Autodesk Inventor part; units mm, degrees
ref_plane "YZ Plane" through (0, 0, 0) normal (1, 0, 0) x (0, 1, 0)
ref_plane "XZ Plane" through (0, 0, 0) normal (0, 1, 0) x (-1, 0, 0)
ref_plane "XY Plane" through (0, 0, 0) normal (0, 0, 1) x (1, 0, 0)
sketch "Boceto1" plane through (0, 0, 0) normal (0, 0, 1) x (1, 0, 0)
  line L0 (0, 71.5) -> (84.4, 71.5)
  line L1 (0, 0) -> (4.5, 0)
  line L2 (62.2, 0) -> (62.2, 35)
  line L3 (62.2, 35) -> (112.2, 35)
  line L4 (112.2, 35) -> (112.2, 0)
  line L5 (84.4, 58.5) -> (84.4, 71.5)
  line L6 (84.4, 58.5) -> (0, 58.5)
  line L7 (87.2, 35) -> (108.2, 35)
  circle A0 centre (108.2, 46.75) radius 1.65
  circle A1 centre (66.2, 46.75) radius 1.65
  circle A2 centre (31.1, 43.75) radius 3
  circle A3 centre (178.7, 0) radius 2.5
  circle A4 centre (68.5, 81.35) radius 1.65
  line L8 (0, 90) -> (105.7, 90)
  arc A5 (120.7782, 83.1308) -> (105.7, 90) centre (105.672, 69.9553) ccw
  line L9 (200, 0) -> (200, 30.4)
  arc A6 (200, 30.4) -> (192, 38.4) centre (192, 30.4) ccw
  arc A7 (120.7782, 83.1308) -> (192, 38.4) centre (202.3119, 133.8853) ccw
  line L10 (4.5, 80.75) -> (4.5, 85.3)
  line L11 (4.5, 85.3) -> (0, 82.7)
  line L12 (4.5, 80.75) -> (4.5, 76.2)
  line L13 (4.5, 76.2) -> (0, 78.8)
  line L14 (0, 90) -> (0, 82.7)
  line L15 (0, 58.5) -> (0, 53.5)
  line L16 (0, 48.4) -> (0, 46.75)
  line L17 (0, 78.8) -> (0, 71.5)
  line L18 (0, 58.5) -> (0, 53.5)
  line L19 (0, 53.5) -> (0, 48.4)
  line L20 (0, 58.5) -> (0, 37.5)
  line L21 (9.1, 34.95) -> (9.1, 41.75)
  line L22 (9.1, 41.75) -> (0, 37.5)
  line L23 (9.1, 34.95) -> (9.1, 28.15)
  line L24 (9.1, 28.15) -> (0, 32.4)
  line L25 (0, 0) -> (0, 32.4)
  line L26 (0, 37.5) -> (0, 46.75)
  line L27 (0, -71.5) -> (84.4, -71.5)
  line L28 (62.2, 0) -> (62.2, -35)
  line L29 (62.2, -35) -> (112.2, -35)
  line L30 (112.2, -35) -> (112.2, 0)
  line L31 (84.4, -58.5) -> (84.4, -71.5)
  line L32 (84.4, -58.5) -> (0, -58.5)
  line L33 (87.2, -35) -> (108.2, -35)
  circle A8 centre (108.2, -46.75) radius 1.65
  circle A9 centre (66.2, -46.75) radius 1.65
  circle A10 centre (31.1, -43.75) radius 3
  circle A11 centre (178.7, 0) radius 2.5
  circle A12 centre (68.5, -81.35) radius 1.65
  line L34 (0, -90) -> (105.7, -90)
  arc A13 (105.7, -90) -> (120.7782, -83.1308) centre (105.672, -69.9553) ccw
  line L35 (200, 0) -> (200, -30.4)
  arc A14 (192, -38.4) -> (200, -30.4) centre (192, -30.4) ccw
  arc A15 (192, -38.4) -> (120.7782, -83.1308) centre (202.3119, -133.8853) ccw
  line L36 (4.5, -80.75) -> (4.5, -85.3)
  line L37 (4.5, -85.3) -> (0, -82.7)
  line L38 (4.5, -80.75) -> (4.5, -76.2)
  line L39 (4.5, -76.2) -> (0, -78.8)
  line L40 (0, -90) -> (0, -82.7)
  line L41 (0, -58.5) -> (0, -53.5)
  line L42 (0, -48.4) -> (0, -46.75)
  line L43 (0, -78.8) -> (0, -71.5)
  line L44 (0, -58.5) -> (0, -53.5)
  line L45 (0, -53.5) -> (0, -48.4)
  line L46 (0, -58.5) -> (0, -37.5)
  line L47 (9.1, -34.95) -> (9.1, -41.75)
  line L48 (9.1, -41.75) -> (0, -37.5)
  line L49 (9.1, -34.95) -> (9.1, -28.15)
  line L50 (9.1, -28.15) -> (0, -32.4)
  line L51 (0, 0) -> (0, -32.4)
  line L52 (0, -37.5) -> (0, -46.75)
  line L53 (261.8168, 58.5) -> (321.3628, 58.5)
  line L54 (321.3628, 58.5) -> (321.3628, -17.5)
  line L55 (321.3628, -17.5) -> (261.8168, -17.5)
  line L56 (261.8168, -17.5) -> (261.8168, 58.5)
sketch "Boceto3" plane through (0, 0, 0) normal (0, 0, 1) x (1, 0, 0)
  line L0 (-258.9506, 92.2639) -> (-258.9506, 96.8139)
  line L1 (-258.9506, 96.8139) -> (-263.4506, 94.2139)
  line L2 (-258.9506, 92.2639) -> (-258.9506, 87.7139)
  line L3 (-258.9506, 87.7139) -> (-263.4506, 90.3139)
  line L4 (-263.4506, 101.5139) -> (-263.4506, 94.2139)
  line L5 (-263.4506, 70.0139) -> (-263.4506, 65.0139)
  line L6 (-263.4506, 59.9139) -> (-263.4506, 58.2639)
  line L7 (-263.4506, 90.3139) -> (-263.4506, 83.0139)
  line L8 (-263.4506, 70.0139) -> (-263.4506, 65.0139)
  line L9 (-263.4506, 65.0139) -> (-263.4506, 59.9139)
  line L10 (-263.4506, 70.0139) -> (-263.4506, 49.0139)
  line L11 (-254.3506, 46.4639) -> (-254.3506, 53.2639)
  line L12 (-254.3506, 53.2639) -> (-263.4506, 49.0139)
  line L13 (-254.3506, 46.4639) -> (-254.3506, 39.6639)
  line L14 (-254.3506, 39.6639) -> (-263.4506, 43.9139)
  line L15 (-263.4506, 11.5139) -> (-263.4506, 43.9139)
  line L16 (-263.4506, 49.0139) -> (-263.4506, 58.2639)
  line L17 (-263.4506, 83.0139) -> (-322.4506, 83.0139)
  line L18 (-263.4506, 83.0139) -> (-322.4506, 83.0139)
  line L19 (-263.4506, 70.0139) -> (-322.4506, 70.0139)
  line L20 (-322.4506, 70.0139) -> (-322.4506, 83.0139)
  circle A0 centre (-322.4506, 55.4139) radius 3
  line L21 (-350.4506, 83.0139) -> (-350.4506, 93.5139)
  circle A1 centre (-272.1006, 92.8639) radius 1.65
  line L22 (-342.4506, 101.5139) -> (-263.4506, 101.5139)
  line L23 (-373.8506, 11.5139) -> (-373.8506, 24.6339)
  arc A2 (-368.1081, 32.3088) -> (-373.8506, 24.6339) centre (-365.8506, 24.6339) ccw
  arc A3 (-342.4506, 101.5139) -> (-350.4506, 93.5139) centre (-342.4506, 93.5139) ccw
  arc A4 (-368.1081, 32.3088) -> (-350.4675, 52.85) centre (-376.4854, 57.3485) ccw
  line L24 (-350.4506, 83.0139) -> (-350.4506, 53.0604)
  arc A5 (-350.4675, 52.85) -> (-350.4506, 53.0604) centre (-357.2375, 53.5013) ccw
  line L25 (-258.9506, -69.2361) -> (-258.9506, -73.7861)
  line L26 (-258.9506, -73.7861) -> (-263.4506, -71.1861)
  line L27 (-258.9506, -69.2361) -> (-258.9506, -64.6861)
  line L28 (-258.9506, -64.6861) -> (-263.4506, -67.2861)
  line L29 (-263.4506, -78.4861) -> (-263.4506, -71.1861)
  line L30 (-263.4506, -46.9861) -> (-263.4506, -41.9861)
  line L31 (-263.4506, -36.8861) -> (-263.4506, -35.2361)
  line L32 (-263.4506, -67.2861) -> (-263.4506, -59.9861)
  line L33 (-263.4506, -46.9861) -> (-263.4506, -41.9861)
  line L34 (-263.4506, -41.9861) -> (-263.4506, -36.8861)
  line L35 (-263.4506, -46.9861) -> (-263.4506, -25.9861)
  line L36 (-254.3506, -23.4361) -> (-254.3506, -30.2361)
  line L37 (-254.3506, -30.2361) -> (-263.4506, -25.9861)
  line L38 (-254.3506, -23.4361) -> (-254.3506, -16.6361)
  line L39 (-254.3506, -16.6361) -> (-263.4506, -20.8861)
  line L40 (-263.4506, 11.5139) -> (-263.4506, -20.8861)
  line L41 (-263.4506, -25.9861) -> (-263.4506, -35.2361)
  line L42 (-263.4506, -59.9861) -> (-322.4506, -59.9861)
  line L43 (-263.4506, -59.9861) -> (-322.4506, -59.9861)
  line L44 (-263.4506, -46.9861) -> (-322.4506, -46.9861)
  line L45 (-322.4506, -46.9861) -> (-322.4506, -59.9861)
  circle A6 centre (-322.4506, -32.3861) radius 3
  line L46 (-350.4506, -59.9861) -> (-350.4506, -70.4861)
  circle A7 centre (-272.1006, -69.8361) radius 1.65
  line L47 (-342.4506, -78.4861) -> (-263.4506, -78.4861)
  line L48 (-373.8506, 11.5139) -> (-373.8506, -1.6061)
  arc A8 (-373.8506, -1.6061) -> (-368.1081, -9.2809) centre (-365.8506, -1.6061) ccw
  arc A9 (-350.4506, -70.4861) -> (-342.4506, -78.4861) centre (-342.4506, -70.4861) ccw
  arc A10 (-350.4675, -29.8221) -> (-368.1081, -9.2809) centre (-376.4854, -34.3207) ccw
  line L49 (-350.4506, -59.9861) -> (-350.4506, -30.0325)
  arc A11 (-350.4506, -30.0325) -> (-350.4675, -29.8221) centre (-357.2375, -30.4734) ccw
  point P0 (0, 0)
sketch "Boceto4" plane through (0, 0, 0) normal (0, 0, 1) x (1, 0, 0)
  line L0 (-279.0503, -82.5554) -> (-279.0503, -78.0054)
  line L1 (-279.0503, -78.0054) -> (-283.5503, -80.6054)
  line L2 (-279.0503, -82.5554) -> (-279.0503, -87.1054)
  line L3 (-279.0503, -87.1054) -> (-283.5503, -84.5054)
  line L4 (-283.5503, -73.3054) -> (-283.5503, -80.6054)
  line L5 (-283.5503, -104.8054) -> (-283.5503, -109.8054)
  line L6 (-283.5503, -114.9054) -> (-283.5503, -116.5554)
  line L7 (-283.5503, -84.5054) -> (-283.5503, -91.8054)
  line L8 (-283.5503, -104.8054) -> (-283.5503, -109.8054)
  line L9 (-283.5503, -109.8054) -> (-283.5503, -114.9054)
  line L10 (-283.5503, -104.8054) -> (-283.5503, -125.8054)
  line L11 (-274.4503, -128.3554) -> (-274.4503, -121.5554)
  line L12 (-274.4503, -121.5554) -> (-283.5503, -125.8054)
  line L13 (-274.4503, -128.3554) -> (-274.4503, -135.1554)
  line L14 (-274.4503, -135.1554) -> (-283.5503, -130.9054)
  line L15 (-283.5503, -163.3054) -> (-283.5503, -130.9054)
  line L16 (-283.5503, -125.8054) -> (-283.5503, -116.5554)
  line L17 (-393.9503, -163.3054) -> (-283.5503, -163.3054)
  line L18 (-283.5503, -91.8054) -> (-342.5503, -91.8054)
  line L19 (-283.5503, -91.8054) -> (-342.5503, -91.8054)
  line L20 (-283.5503, -104.8054) -> (-342.5503, -104.8054)
  line L21 (-342.5503, -104.8054) -> (-342.5503, -91.8054)
  circle A0 centre (-342.5503, -119.4054) radius 3
  line L22 (-370.5503, -91.8054) -> (-370.5503, -81.3054)
  circle A1 centre (-292.2003, -81.9554) radius 1.65
  line L23 (-362.5503, -73.3054) -> (-283.5503, -73.3054)
  line L24 (-393.9503, -163.3054) -> (-393.9503, -150.1854)
  arc A2 (-388.2078, -142.5105) -> (-393.9503, -150.1854) centre (-385.9503, -150.1854) ccw
  arc A3 (-362.5503, -73.3054) -> (-370.5503, -81.3054) centre (-362.5503, -81.3054) ccw
  arc A4 (-388.2078, -142.5105) -> (-370.5672, -121.9694) centre (-396.5851, -117.4708) ccw
  line L25 (-370.5503, -91.8054) -> (-370.5503, -121.7589)
  arc A5 (-370.5672, -121.9694) -> (-370.5503, -121.7589) centre (-377.3372, -121.318) ccw
  point P0 (0, 0)
  point P1 (89.2704, -12.3046)
  dimension "d61" = 13.12
  dimension "d62" = 8
extrude "Extrusión2" add sketch "Boceto3" along normal blind 6.35
fillet "Empalme3" radius 0.01 22 edges at (-348.1074, 99.1708, 6.35) (-350.4506, 88.2639, 6.35) (-302.9506, 101.5139, 6.35) (-356.4543, 40.1461, 6.35) (-373.8506, 18.0739, 6.35) (-372.256, -6.3988, 6.35) (-372.256, 29.4266, 6.35) (-356.4543, -17.1182, 6.35) (-348.1074, -76.1429, 6.35) (-302.9506, -78.4861, 6.35) (-350.4506, -45.0093, 6.35) (-348.1074, 99.1708, 0) (-350.4506, 88.2639, 0) (-302.9506, 101.5139, 0) (-356.4543, 40.1461, 0) (-373.8506, 18.0739, 0) (-372.256, -6.3988, 0) (-372.256, 29.4266, 0) (-356.4543, -17.1182, 0) (-348.1074, -76.1429, 0) (-302.9506, -78.4861, 0) (-350.4506, -45.0093, 0)
equation "\"Radio_pliegue\" = Grosor"
equation "\"Anchura_desahogo_plegado\" = Grosor"
equation "\"Profundidad_desahogo_plegado\" = 0.5 * Grosor"
equation "\"Tamaño_destalonado\" = 4 * Grosor"
equation "\"Remanente_mínimo\" = 2 * Grosor"
equation "\"Radiodetransición\" = Radio_pliegue"
equation "\"Tamaño_de_radio_de_Jacobi\" = Radio_pliegue"
equation "\"TamañoSeparación\" = Grosor"
properties part number "tmr"
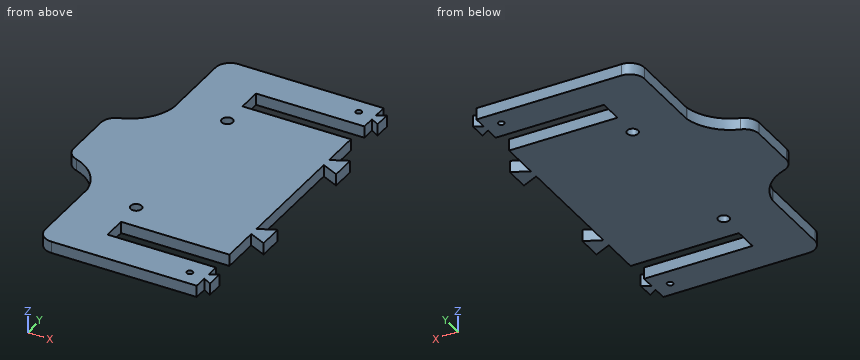
Check sheet for the modelled part. Datum: model origin and axes. Units: mm. Give positions to 0.01 mm unless a question says otherwise; leave off trailing zeros. Answer in a Markdown table with one row per item.
1) Depth check by flat-ended pin: pin 1 (3 mm diameter, centred on y = -70.5, z = 3, fed in from +X); pin 2 (2 mm diameter, centred on x = -350, z = 5, fed in from +Y); pin 3 (2 mm diameter, centred on x = -361, z = 3, fed in from +Y). Enter the tip coordinate at first touch or a pass-through.
Solutions:
| item | result |
|---|---|
| pin 1 | stops at x = -258.95 |
| pin 2 | stops at y = 98.11 |
| pin 3 | stops at y = 36.72 |
2) Cross-section at A-A (x = -296). Count the separate pieces of the cut face and the enclosed holes in it, plus the area to 3 significant figures.
Solutions:
| item | result |
|---|---|
| separate pieces | 3 |
| enclosed holes | 0 |
| area | 978 mm^2 |
3) Thickness scan on line 1 (Y direction, x = -278, z = 5); line 2 (Y direction, x = -260, z = 3); line 3 (X direction, y = 62, z = 1.75). Record the ranges inside material, lowest first.
Solutions:
| item | result |
|---|---|
| line 1 | y = -78.49 to -59.99, -46.99 to 70.01, 83.01 to 101.51 |
| line 2 | y = -73.18 to -65.29, -27.6 to -19.27, 42.3 to 50.63, 88.32 to 96.21 |
| line 3 | x = -350.45 to -263.45 |
